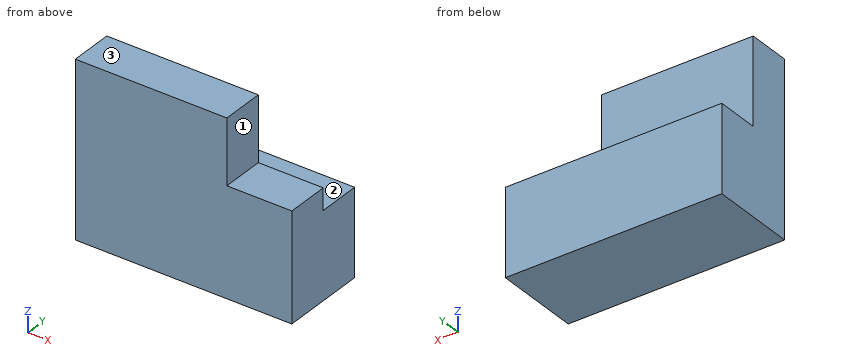
from build123d import *

# Parameters (mm, degrees)
F0_W     = 50
F0_H     = 40
F1_DEPTH = 10
F2_W     = 15
F2_H     = 15
F3_DEPTH = 10.001
F4_W     = 50
F4_H     = 10
F5_DEPTH = 20


with BuildPart() as f1:
    # F0 (on Front) → F1 (new body)
    with BuildSketch(Plane.XZ):
        Rectangle(F0_W, F0_H)
    extrude(amount=F1_DEPTH)

    # F2 (on Front) → F3 (cut, through all)
    with BuildSketch(Plane.XZ):
        with Locations((17.5, 12.5)):
            Rectangle(F2_W, F2_H)
    extrude(amount=F3_DEPTH, mode=Mode.SUBTRACT)

    # F4 (on Top) → F5 (join)
    with BuildSketch(Plane.XY):
        with Locations((0, 5)):
            Rectangle(F4_W, F4_H)
    extrude(amount=-F5_DEPTH)


solid = f1.part
Could you check a few things on this model? Use its own coordinates, in mm. Face numbers are marked on the shaded views. A direction names the side the tool comes from. Give positions to 0.01 mm unless a question says otherwise; leave off trailing zeros. Order: outer loops, then holes, each group sorted by start corner. A loop starts at its lowest first (then second) coordinate and runs counter-clockwise, first axis right, second up.
Item 1: If we section it at D-D, the plane y = 2: Write out the boundary of the cut face in (x, z), plus the area to 3 significant figures.
Item 2: I'm going to push flat-ended pins straight in: pin 1 (10 mm diameter, centred on x = 2, z = 6, fed in from +Y); pin 2 (8 mm diameter, centred on y = -3.5, z = 14, fed in from +X); pin 3 (8 mm diameter, centred on x = 19.5, y = -6, fed in from +Z). Where does each tip first touch, or does it pass through?
Item 3: If we section it at B-B, the plane x = 18: Write out the boundary of the cut face in (y, z), plus the area to 3 significant figures.
Item 4: I need wall thicknesses on line 1 (Y direction, x = -12.5, z = 12); line 2 (X direction, y = -2, z = 8); line 3 (Z direction, x = -19, y = 4). Which ranges of each line are inside material? Lowest first, please.
Item 5: For the marked faces 1, 2 and 3, which set-ups out of +Z, -Z, +X, -X, +Y, -Y let a thin tool reach every point of the face, with its end or its side?
Item 6: If we section it at C-C, the plane z = 3: Write out the boundary of the cut face in (x, y).
Item 7: If we section it at A-A, the plane y = -2.25: Write out the boundary of the cut face in (x, z), plus the area to 4 significant figures.
Values:
1. outline: (-25, -20) - (25, -20) - (25, 0) - (-25, 0) - close
1. area: 1,000 mm2
2. pin 1: stops at y = 0
2. pin 2: stops at x = 10
2. pin 3: stops at z = 5
3. outline: (-10, -20) - (10, -20) - (10, 0) - (0, 0) - (0, 5) - (-10, 5) - close
3. area: 450 mm2
4. line 1: y = -10 to 0
4. line 2: x = -25 to 10
4. line 3: z = -20 to 0
5. face 1: +Z, +X, +Y, -Y
5. face 2: +Z, +X, -X, +Y
5. face 3: +Z, +X, -X, +Y, -Y
6. outline: (-25, -10) - (25, -10) - (25, 0) - (-25, 0) - close
7. outline: (-25, -20) - (25, -20) - (25, 5) - (10, 5) - (10, 20) - (-25, 20) - close
7. area: 1,775 mm2
